from build123d import *

# Parameters (mm, degrees)
BOSS_EXTRUDE1_DEPTH = 5.08
SKETCH3_R           = 1.905
CUT_EXTRUDE1_DEPTH  = 6.08
SKETCH4_R           = 1.905
SKETCH4_R_2         = 2.286
CUT_EXTRUDE2_DEPTH  = 6.08
CUT_EXTRUDE3_DEPTH  = 6.08
SKETCH6_R           = 15.494
SKETCH6_R_2         = 1.7
CUT_EXTRUDE4_DEPTH  = 6.08
SKETCH7_W           = 55.88
SKETCH7_H           = 73.66
CUT_EXTRUDE5_DEPTH  = 6.08
SKETCH8_W           = 5.838418679
SKETCH8_H           = 5.514062087
CUT_EXTRUDE6_DEPTH  = 6.08
CUT_EXTRUDE7_DEPTH  = 6.08
SKETCH12_W          = 10.16
SKETCH12_H          = 7.62
CUT_EXTRUDE8_DEPTH  = 6.08
SKETCH13_W          = 41.91
SKETCH13_H          = 15.24
CUT_EXTRUDE9_DEPTH  = 2.54


with BuildPart() as part:
    # Sketch1 → Boss-Extrude1 (new body)
    with BuildSketch(Plane(origin=(0, 0, 0), x_dir=(1, 0, 0), z_dir=(0, 1, 0))):
        Polygon((-15.621, -53.34), (15.621, -53.34), (88.265, -53.34), (88.265, 53.34), (-88.265, 53.34), (-88.265, -53.34), align=None)
    extrude(amount=BOSS_EXTRUDE1_DEPTH)

    # Sketch3 → Cut-Extrude1 (cut, through all)
    with BuildSketch(Plane(origin=(0, 5.08, 0), x_dir=(1, 0, 0), z_dir=(0, 1, 0))):
        with Locations((-81.915, 46.99)):
            Circle(SKETCH3_R)
    extrude(amount=-CUT_EXTRUDE1_DEPTH, mode=Mode.SUBTRACT)

    # Sketch4 → Cut-Extrude2 (cut, through all)
    with BuildSketch(Plane(origin=(0, 5.08, 0), x_dir=(1, 0, 0), z_dir=(0, 1, 0))):
        with Locations((81.915, 46.99)):
            Circle(SKETCH4_R)
        with Locations((-81.915, -46.99)):
            Circle(SKETCH4_R)
        with Locations((81.915, -46.99)):
            Circle(SKETCH4_R)
        with Locations((23.495, 40.64)):
            Circle(SKETCH4_R_2)
        with Locations((-23.495, 40.64)):
            Circle(SKETCH4_R_2)
    extrude(amount=-CUT_EXTRUDE2_DEPTH, mode=Mode.SUBTRACT)

    # Sketch5 → Cut-Extrude3 (cut, through all)
    with BuildSketch(Plane.XZ):
        Polygon((-2.54, 27.94), (-2.54, 5.969), (11.811, 5.969), (11.811, 0.127), (14.859, 0.127), (14.859, 5.969), (33.02, 5.969), (33.02, 29.21), (33.02, 31.75), (26.67, 31.75), (26.67, 27.94), (25.80916534, 27.94), (14.859, 27.94), (14.859, 33.782), (11.811, 33.782), (11.811, 27.94), align=None)
    extrude(amount=-CUT_EXTRUDE3_DEPTH, mode=Mode.SUBTRACT)

    # Sketch6 → Cut-Extrude4 (cut, through all)
    with BuildSketch(Plane(origin=(0, 5.08, 0), x_dir=(1, 0, 0), z_dir=(0, 1, 0))):
        with Locations((60.071, 25.146)):
            Circle(SKETCH6_R)
        with Locations((39.9778, 25.146)):
            Circle(SKETCH6_R_2)
        with Locations((80.1642, 25.146)):
            Circle(SKETCH6_R_2)
    extrude(amount=-CUT_EXTRUDE4_DEPTH, mode=Mode.SUBTRACT)

    # Sketch7 → Cut-Extrude5 (cut, through all)
    with BuildSketch(Plane(origin=(0, 5.08, 0), x_dir=(1, 0, 0), z_dir=(0, 1, 0))):
        with Locations((-52.705, -3.81)):
            Rectangle(SKETCH7_W, SKETCH7_H)
    extrude(amount=-CUT_EXTRUDE5_DEPTH, mode=Mode.SUBTRACT)

    # Sketch8 → Cut-Extrude6 (cut, through all)
    with BuildSketch(Plane(origin=(0, 5.08, 0), x_dir=(1, 0, 0), z_dir=(0, 1, 0))):
        with Locations((52.991758435, 3.486833379)):
            Rectangle(SKETCH8_W, SKETCH8_H)
    extrude(amount=-CUT_EXTRUDE6_DEPTH, mode=Mode.SUBTRACT)

    # Sketch11 → Cut-Extrude7 (cut, through all)
    with BuildSketch(Plane.XZ):
        Polygon((29.845, 31.75), (51.435, 31.75), (51.435, 41.91), (29.845, 41.91), (22.225, 41.91), (22.225, 34.29), (29.845, 34.29), align=None)
    extrude(amount=-CUT_EXTRUDE7_DEPTH, mode=Mode.SUBTRACT)

    # Sketch12 → Cut-Extrude8 (cut, through all)
    with BuildSketch(Plane.XZ):
        with Locations((-10.16, 38.1)):
            Rectangle(SKETCH12_W, SKETCH12_H)
    extrude(amount=-CUT_EXTRUDE8_DEPTH, mode=Mode.SUBTRACT)

    # Sketch13 → Cut-Extrude9 (cut)
    with BuildSketch(Plane(origin=(0, 5.08, 0), x_dir=(1, 0, 0), z_dir=(0, 1, 0))):
        with Locations((14.605, -39.37)):
            Rectangle(SKETCH13_W, SKETCH13_H)
    extrude(amount=-CUT_EXTRUDE9_DEPTH, mode=Mode.SUBTRACT)


solid = part.part
Build history of the part. All positions in model axes, mm. Round coordinates to 2 decimals unless told otherwise and drop trailing zeros. Loops run counter-clockwise (first coordinate to the right, second up) from the corner with the lowest first, then second, coordinate; pieces in that order, holes last. Notation, with made-up numbers: (67.5, -36) -> (101.5, -36) arc R9 ccw to (101.5, -27) -> close; hole circle Ø11 at (-4, -16.75). An arc over 180 degrees is marked (long way). One line per item, written item: value. Start each with the question number.
Q1. Drop a flat-ended pin along its axis: pin 1 Ø4 at (x, z) = (-23.495, -40.64) entering from -Y. Give the stop position or say it passes through.
Q2. Cut at B-B on x = -32. List the corners of the cut face in (y, z), plus the area to 3 significant figures.
Q3. Cut at D-D on y = 1.5. Count the separate pieces of the cut face and the enclosed holes in it, plus the area to 3 significant figures.
Q4. Two-plate mould, pull along Z, no slides. Class faces 1 (the face through (55.911, 3, -3)), 2 (the face through (88.265, 3, 1)), 3 (the face through (1, 3, -53.34)): released by +Z, released by -Z, zero draft, split by the parting line, or undercut.
Q5. Cut at A-A on z = -46.99. List the corners of the cut face in (x, y) (3 decimals), plus the area to 3 significant figures.
Q6. Probe line 1 along X through (y, z) = (0.45, 3) (3 decimals); line 2 along X through (y, z) = (3.45, -46.99) (3 decimals); line 3 along X through (y, z) = (2, 32) (3 decimals). List the from-to ranges inside material, lowest first.
Q7. Cut at C-C on z = 24. List the corners of the cut face in (x, y) (3 decimals), plus the area to 3 significant figures.
Computed:
1. pin 1: through
2. outline: (0, -53.34) -> (5.08, -53.34) -> (5.08, -33.02) -> (0, -33.02) -> close; (0, 40.64) -> (5.08, 40.64) -> (5.08, 53.34) -> (0, 53.34) -> close
2. area: 168 mm²
3. separate pieces: 1
3. enclosed holes: 13
3. area: 12,600 mm²
4. face 1: undercut
4. face 2: zero draft
4. face 3: released by -Z
5. outline: (-88.265, 0) -> (-83.82, 0) -> (-83.82, 5.08) -> (-88.265, 5.08) -> close; (-80.01, 0) -> (80.01, 0) -> (80.01, 5.08) -> (-80.01, 5.08) -> close; (83.82, 0) -> (88.265, 0) -> (88.265, 5.08) -> (83.82, 5.08) -> close
5. area: 858 mm²
6. line 1: -88.265 to -80.645, -24.765 to 11.811, 14.859 to 88.265
6. line 2: -88.265 to -83.82, -80.01 to 80.01, 83.82 to 88.265
6. line 3: -88.265 to -80.645, -24.765 to 11.811, 14.859 to 29.845, 51.435 to 88.265
7. outline: (-88.265, 0) -> (-80.645, 0) -> (-80.645, 5.08) -> (-88.265, 5.08) -> close; (-24.765, 0) -> (-2.54, 0) -> (-2.54, 5.08) -> (-24.765, 5.08) -> close; (33.02, 0) -> (88.265, 0) -> (88.265, 5.08) -> (33.02, 5.08) -> close
7. area: 432 mm²
